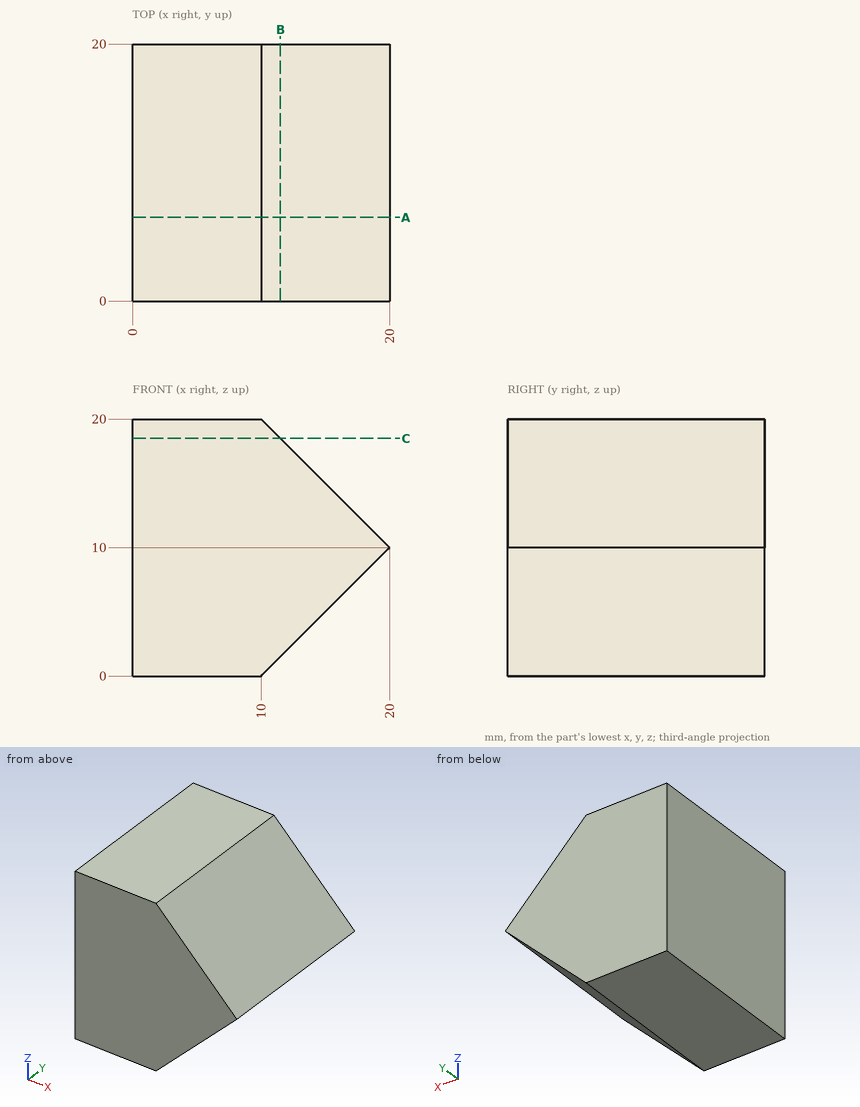
Geometry: see drawing. Coordinates: mm, zero at the bounding-box minimum. Give positions to 0.01 mm unless a question says otherwise; leave off trailing zeros. Order: outer loops, then holes, each group sorted by start corner. A loop starts at its lowest first (then second) coordinate and runs counter-clockwise, first axis right, second up.
1. Cut plane C-C (z = 18.5). Return loops of the section in (x, y), and give its area (3 significant figures).
Computed:
outline: (0, 0) - (11.5, 0) - (11.5, 20) - (0, 20) - close
area: 230 mm2
2. Cut plane B-B (x = 11.5). Return loops of the section in (y, z).
Computed:
outline: (0, 1.5) - (20, 1.5) - (20, 18.5) - (0, 18.5) - close
3. Line query: probe 1 along Z at (x, y) = (18.5, 10.5); probe 2 along Z at (x, y) = (17.25, 14.5); probe 3 along X at (y, z) = (10.5, 3). Output: solid intervals per line, ascending.
Computed:
probe 1: z = 8.5 to 11.5
probe 2: z = 7.25 to 12.75
probe 3: x = 0 to 13
4. Cut plane A-A (y = 6.5). Return loops of the section in (x, z), and give its area (3 significant figures).
Computed:
outline: (0, 0) - (10, 0) - (20, 10) - (10, 20) - (0, 20) - close
area: 300 mm2
5. Pin query (flat end, axial travel): pin 1 Ø5 at (x, y) = (13, 8.5) entering from -Z; pin 2 Ø1.5 at (x, y) = (12.5, 7) entering from +Z; pin 3 Ø2 at (x, y) = (18, 3) entering from -Z. Return the tip coordinate at first contact, or that it passes through.
Computed:
pin 1: stops at z = 0.5
pin 2: stops at z = 18.25
pin 3: stops at z = 7
